Read the model definition and answer for the solid it produces. Units are mm, in the model's axes. Coordinates: 2 decimals unless noted, no trailing zeros. Write each loop counter-clockwise with the first axis right and the second up, starting at its lowest first coordinate (ties: lowest second). Pieces come first, ordered by that corner, then holes. Notation, with made-up numbers: (29, 44.5) -> (81, 44.5) arc R17 cw to (81, 56.5) -> close; hole circle Ø8 at (13, 26). An arc over 180 degrees is marked (long way). Write item = value, one per line. Start each with the question number.
1) Section B-B (z = 4.5) is taken. Count the separate pieces of the cut face and the enclosed holes in it, plus the area to 3 significant figures.
2) Section A-A (x = 26) is taken. Determine the outline of the cut face in (y, z).
3) Find the intervals of material crossed by line 1 along Y through (x, z) = (13, 2.25); line 2 along Y through (x, z) = (32.5, 6); line 3 along Y through (x, z) = (5, 2.5), in increasing order. Write a range as from..to.
4) For a pull along Y with two mould halves and no side action, classify faces 1 (the face through (2.835, 26.127, 3.131)), 2 (the face through (0, 18, 3)), 3 (the face through (19, 35, 3)), 4 (the face through (0.57, 0.6, 3.13)) as released by +Y, released by -Y, zero draft, split by the parting line, or undercut.
from build123d import *

# Parameters (mm, degrees)
SKETCH1_R           = 1.65
SKETCH1_R_2         = 2.2
SKETCH1_R_3         = 2.1
SKETCH1_R_4         = 2.75
SKETCH1_R_5         = 1.75
SKETCH1_R_6         = 2.3
SKETCH1_R_7         = 2.85
SKETCH1_R_8         = 2.65
SKETCH1_R_9         = 2
SKETCH1_R_10        = 1.25
SKETCH1_R_11        = 1.35
SKETCH1_R_12        = 1.55
SKETCH1_R_13        = 1.15
BOSS_EXTRUDE1_DEPTH = 6.35


with BuildPart() as part:
    # Sketch1 → Boss-Extrude1 (new body)
    with BuildSketch(Plane.XY):
        with BuildLine():
            Line((2, 0), (38, 0))
            Line((38, 0), (38, 33))
            ThreePointArc((38, 33), (37.414213562, 34.414213562), (36, 35))
            Line((36, 35), (2, 35))
            ThreePointArc((2, 35), (0.585786438, 34.414213562), (0, 33))
            Line((0, 33), (0, 2))
            ThreePointArc((0, 2), (0.585786438, 0.585786438), (2, 0))
        make_face()
        with Locations((8.336360719, 27.737428386)):
            Circle(SKETCH1_R, mode=Mode.SUBTRACT)
        with Locations((27.124645172, 27.737428386)):
            Circle(SKETCH1_R_2, mode=Mode.SUBTRACT)
        with Locations((8.336360719, 14.775034728)):
            Circle(SKETCH1_R_3, mode=Mode.SUBTRACT)
        with Locations((27.124645172, 14.775034728)):
            Circle(SKETCH1_R_4, mode=Mode.SUBTRACT)
        with Locations((13.899554089, 27.737428386)):
            Circle(SKETCH1_R_5, mode=Mode.SUBTRACT)
        with Locations((33.982726189, 27.737428386)):
            Circle(SKETCH1_R_6, mode=Mode.SUBTRACT)
        with Locations((20.195125811, 27.737428386)):
            Circle(SKETCH1_R_3, mode=Mode.SUBTRACT)
        with Locations((3.192799956, 27.737428386)):
            Circle(SKETCH1_R, mode=Mode.SUBTRACT)
        with Locations((33.982726189, 14.775034728)):
            Circle(SKETCH1_R_7, mode=Mode.SUBTRACT)
        with Locations((20.195125811, 14.775034728)):
            Circle(SKETCH1_R_8, mode=Mode.SUBTRACT)
        with Locations((3.192799956, 14.775034728)):
            Circle(SKETCH1_R_9, mode=Mode.SUBTRACT)
        with Locations((13.899554089, 14.775034728)):
            Circle(SKETCH1_R_2, mode=Mode.SUBTRACT)
        with Locations((8.336360719, 5.504307148)):
            Circle(SKETCH1_R_10, mode=Mode.SUBTRACT)
        with Locations((27.124645172, 5.504307148)):
            Circle(SKETCH1_R, mode=Mode.SUBTRACT)
        with Locations((13.899554089, 5.504307148)):
            Circle(SKETCH1_R_11, mode=Mode.SUBTRACT)
        with Locations((33.982726189, 5.504307148)):
            Circle(SKETCH1_R_5, mode=Mode.SUBTRACT)
        with Locations((20.195125811, 5.504307148)):
            Circle(SKETCH1_R_12, mode=Mode.SUBTRACT)
        with Locations((3.192799956, 5.504307148)):
            Circle(SKETCH1_R_13, mode=Mode.SUBTRACT)
    extrude(amount=BOSS_EXTRUDE1_DEPTH)


solid = part.part
Answer key:
q1.separate_pieces = 1
q1.enclosed_holes = 18
q1.area = 1,100 mm^2
q2.outline = (0, 0) -> (4.3, 0) -> (4.3, 6.35) -> (0, 6.35) -> close; (6.71, 0) -> (12.27, 0) -> (12.27, 6.35) -> (6.71, 6.35) -> close; (17.28, 0) -> (25.85, 0) -> (25.85, 6.35) -> (17.28, 6.35) -> close; (29.63, 0) -> (35, 0) -> (35, 6.35) -> (29.63, 6.35) -> close
q3.line_1 = 0..4.5, 6.51..12.77, 16.78..26.24, 29.24..35
q3.line_2 = 0..4.57, 6.43..12.34, 17.21..25.98, 29.5..35
q3.line_3 = 0..13.92, 15.63..35
q4.face_1 = undercut
q4.face_2 = zero draft
q4.face_3 = released by +Y
q4.face_4 = released by -Y
